Geometry: see drawing. Coordinates: mm, zero at the bounding-box minimum. Coordinates: 2 decimals unless noted, no trailing zeros. Order: outer loops, then holes, each group sorted by start corner. A loop starts at its lowest first (then second) coordinate and runs counter-clockwise, first axis right, second up. Notation, with made-up numbers: (-15, 87.5) -> (11, 87.5) arc R11 cw to (11, 107.5) -> close; hole circle Ø3 at (-7.75, 11). An arc over 180 degrees is marked (long way). Use CSV: the item, a comma, the result in double quotes. Start each with the question number.
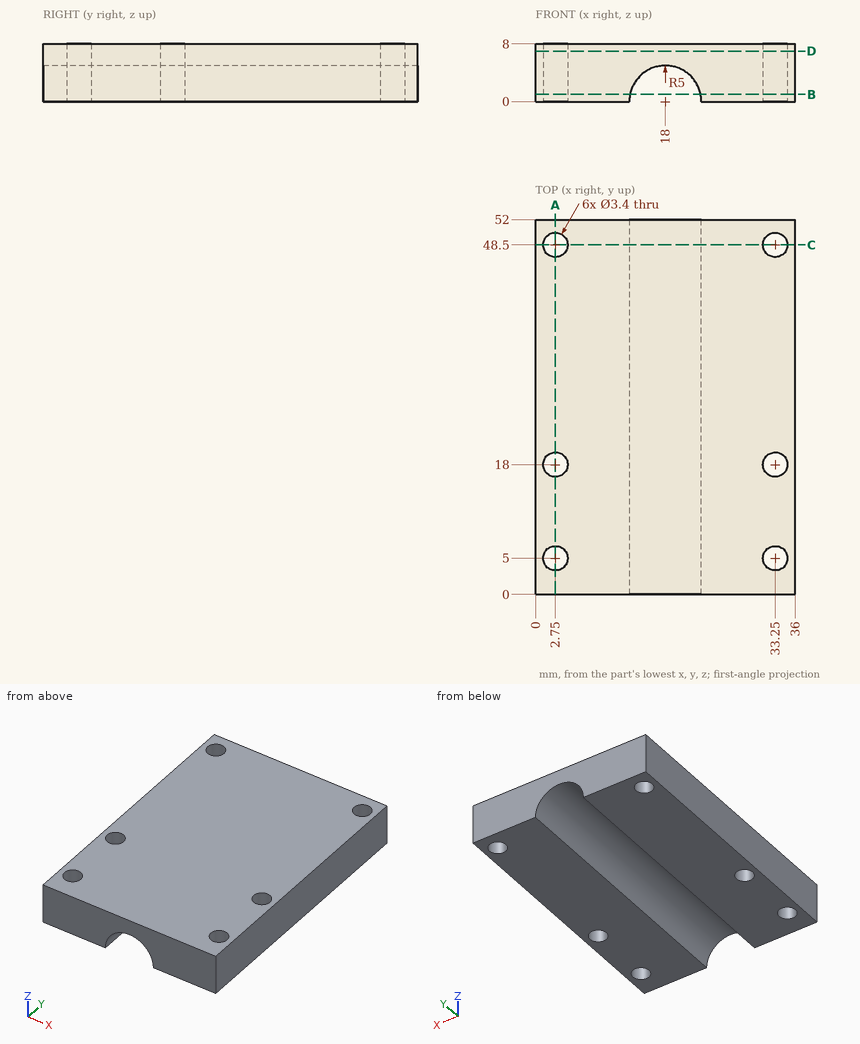
(1) Section D-D (z = 7). Return loops of the section in (x, y).
(2) Section C-C (y = 48.5). Return loops of the section in (x, z), then the cut area to 3 significant figures.
(3) Section B-B (z = 1). Return loops of the section in (x, y).
(4) Section A-A (x = 2.75). Return loops of the section in (y, z).
(5) Line query: line 1 (Y direction, x = 2.75, z = 2.25); line 2 (X direction, y = 16.5, z = 1.5); line 3 (X direction, y = 5.5, z = 1.5). Output: solid intervals per line, ascending. Write a range as from..to.
Check sheet entries:
1,outline,"(0, 0) -> (36, 0) -> (36, 52) -> (0, 52) -> close; hole circle Ø3.4 at (2.75, 5); hole circle Ø3.4 at (2.75, 18); hole circle Ø3.4 at (2.75, 48.5); hole circle Ø3.4 at (33.25, 5); hole circle Ø3.4 at (33.25, 18); hole circle Ø3.4 at (33.25, 48.5)"
2,outline,"(0, 0) -> (1.05, 0) -> (1.05, 8) -> (0, 8) -> close; (4.45, 0) -> (13, 0) arc R5 cw to (23, 0) -> (31.55, 0) -> (31.55, 8) -> (4.45, 8) -> close; (34.95, 0) -> (36, 0) -> (36, 8) -> (34.95, 8) -> close"
2,area,"194 mm^2"
3,outline,"(0, 0) -> (13.1, 0) -> (13.1, 52) -> (0, 52) -> close; (22.9, 0) -> (36, 0) -> (36, 52) -> (22.9, 52) -> close; hole circle Ø3.4 at (2.75, 5); hole circle Ø3.4 at (2.75, 18); hole circle Ø3.4 at (2.75, 48.5); hole circle Ø3.4 at (33.25, 5); hole circle Ø3.4 at (33.25, 18); hole circle Ø3.4 at (33.25, 48.5)"
4,outline,"(0, 0) -> (3.3, 0) -> (3.3, 8) -> (0, 8) -> close; (6.7, 0) -> (16.3, 0) -> (16.3, 8) -> (6.7, 8) -> close; (19.7, 0) -> (46.8, 0) -> (46.8, 8) -> (19.7, 8) -> close; (50.2, 0) -> (52, 0) -> (52, 8) -> (50.2, 8) -> close"
5,line 1,"y = 0..3.3, 6.7..16.3, 19.7..46.8, 50.2..52"
5,line 2,"x = 0..1.95, 3.55..13.23, 22.77..32.45, 34.05..36"
5,line 3,"x = 0..1.13, 4.37..13.23, 22.77..31.63, 34.87..36"
